Could you check a few things on this drawing? It's one solid part, dimensions in mm from its lowest x, y, z. A direction names the side the tool comes from. Give positions to 0.01 mm unless a question says otherwise; leave off trailing zeros. Loops run counter-clockwise (first coordinate to the right, second up) from the corner with the lowest first, then second, coordinate; pieces in that order, holes last. Notation, with made-up numbers: (20.5, -19.75) - (42.5, -19.75) arc R20 cw to (42.5, -13.75) - close; hole circle Ø8 at (19, 59.25). An arc over 180 degrees is marked (long way). Return JSON: item names as keys, results as strings. Group by question number.
(1) If we section it at A-A (y = 19): Please give me the cut outline in (x, z), then the cut area to 3 significant figures.
(2) If we section it at B-B (z = 5.5): Please give me the cut outline in (x, y).
(3) If we mould it in two halves opening along X, with no side actions, what happens to the marked faces 1, 2 and 3? For each: released by +X, released by -X, zero draft, split by the parting line, or undercut.
(4) On a 3-axis mill with a long thin cutter (end or side, diameter ignored), from which of +Z, -Z, +X, -X, +Y, -Y can I reach the whole of each face in a straight line? I mean the marked faces 4, 5, 6, 7 and 8. Say none if no direction works.
(5) If we section it at C-C (x = 23.5): Please give me the cut outline in (y, z).
(6) For P1, Ø4, axis at x = 12.5, z = 5, coming from the +Y side; P2, Ø2.5, axis at x = 16.5, z = 4.5, coming from the -Y side; P3, Ø0.8, axis at x = 13.5, z = 9, coming from the -Y side, each with a flat end and sliding along its axis, tell me the tip position at first contact or that it passes through.
(7) I need wall thicknesses on probe 1 along X at (y, z) = (9.5, 4.5); probe 2 along Y at (x, z) = (11, 7.25); probe 3 along Y at (x, z) = (23.75, 3.75). Which ranges of each line are inside material? Lowest first, please. Write a range as [from, to].
(8) If we section it at D-D (y = 6.5): Please give me the cut outline in (x, z), then the cut area to 3 significant figures.
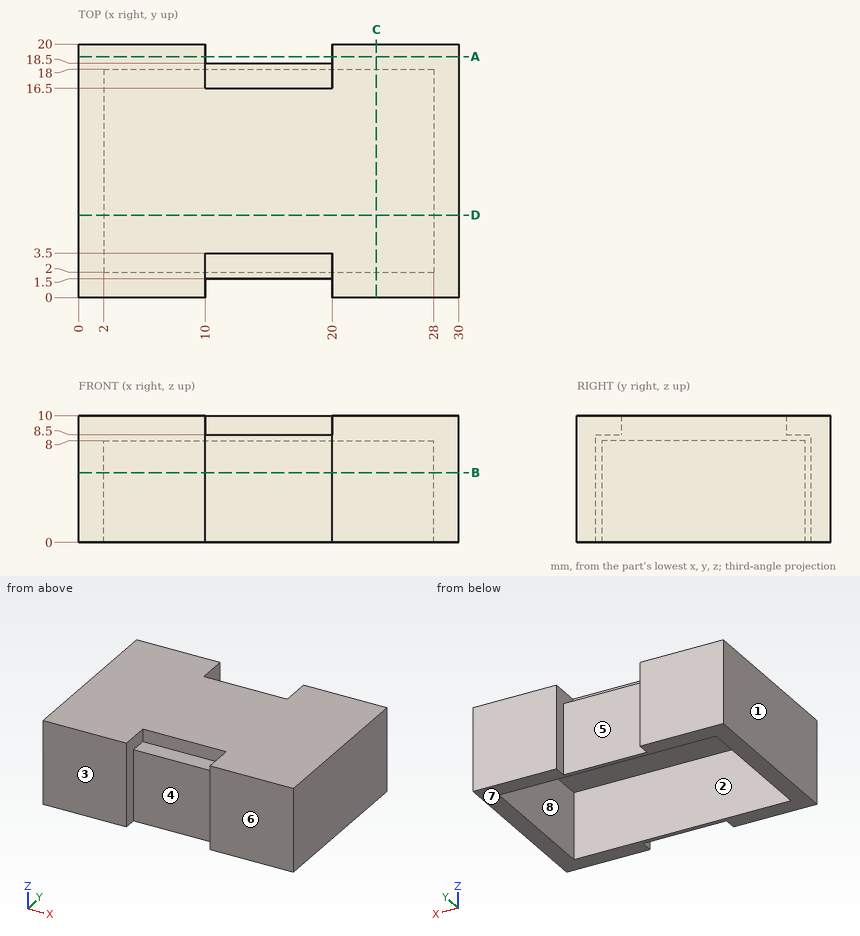
Values:
{
 "1": {"outline": "(0, 0) - (10, 0) - (10, 10) - (0, 10) - close; (20, 0) - (30, 0) - (30, 10) - (20, 10) - close", "area": "200 mm2"},
 "2": {"outline": "(0, 0) - (10, 0) - (10, 1.5) - (20, 1.5) - (20, 0) - (30, 0) - (30, 20) - (20, 20) - (20, 18.5) - (10, 18.5) - (10, 20) - (0, 20) - close; hole (2, 2) - (28, 2) - (28, 18) - (2, 18) - close"},
 "3": {"face 1": "released by -X", "face 2": "undercut", "face 3": "zero draft"},
 "4": {"face 4": "+Z, -Z, -Y", "face 5": "+Z, -Z, +Y", "face 6": "+Z, -Z, +X, -X, -Y", "face 7": "-Z, +X, -X, +Y, -Y", "face 8": "-Z"},
 "5": {"outline": "(0, 0) - (2, 0) - (2, 8) - (18, 8) - (18, 0) - (20, 0) - (20, 10) - (0, 10) - close"},
 "6": {"P1": "y = 18.5", "P2": "y = 1.5", "P3": "y = 3.5"},
 "7": {"probe 1": "[0, 2], [28, 30]", "probe 2": "[1.5, 2], [18, 18.5]", "probe 3": "[0, 2], [18, 20]"},
 "8": {"outline": "(0, 0) - (2, 0) - (2, 8) - (28, 8) - (28, 0) - (30, 0) - (30, 10) - (0, 10) - close", "area": "92.0 mm2"}
}
